For this review, take the finished solid that the model builds, in its own axes (mm). Round coordinates to 2 decimals unless told otherwise and drop trailing zeros. Write each loop counter-clockwise with the first axis right and the second up, starting at its lowest first coordinate (ties: lowest second). Pieces come first, ordered by that corner, then holes. Notation, with made-up numbers: (5, 15.25) - (60, 15.25) arc R27 ccw to (60, 41.25) - close; hole circle Ø3 at (63, -26.5). An arc over 180 degrees is marked (long way). One line per item, written item: value. Start each with the question number.
Q1. Clearance check with flat-ended pins moving along their axes: pin 1 Ø1.5 at (y, z) = (28, 1.5) entering from -X; pin 2 Ø1.5 at (y, z) = (-18, 1) entering from +X; pin 3 Ø0.9 at (y, z) = (79.5, 1.5) entering from -X; pin 4 Ø12 at (x, y) = (-57.5, 5.5) entering from -Z. State where each tip first meets the part, or that it passes through.
Q2. Add section A-A on x = -21. Write out the cut boundary in (y, z).
Q3. For probe 1 along Y at (x, z) = (-22, 0.65); probe 2 along X at (y, z) = (36, 0.7); probe 3 along Y at (x, z) = (23.5, 2.3), list the stretches that pass through material, from the lowest coordinate up.
Q4. Add section C-C on z = 2.15. Give the number of separate pieces and of enclosed holes in the cut face, and give its area (3 significant figures).
Q5. Add section B-B on y = 31.5. Write out the cut boundary in (x, z).
```python
from build123d import *

# Parameters (mm, degrees)
ESQUISSE1_R        = 2.428661445
ESQUISSE1_R_2      = 2.544536974
ESQUISSE1_R_3      = 2.470557968
BOSS_EXTRU_1_DEPTH = 3


with BuildPart() as part:
    # Esquisse1 → Boss.-Extru.1 (new body)
    with BuildSketch(Plane.XY):
        Polygon((-10.741833575, 80.200130208), (19.258166425, 80.200130208), (19.258166425, 77.200130208), (26.258166425, 77.200130208), (26.258166425, 70.200130208), (29.258166425, 70.200130208), (29.258166425, 40.200130208), (26.258166425, 40.200130208), (26.258166425, 20.200130208), (29.258166425, 20.200130208), (29.258166425, -9.799869792), (26.258166425, -9.799869792), (26.258166425, -16.799869792), (19.258166425, -16.799869792), (19.258166425, -19.799869792), (-10.741833575, -19.799869792), (-10.741833575, -16.799869792), (-30.741833575, -16.799869792), (-30.741833575, -19.799869792), (-60.741833575, -19.799869792), (-60.741833575, -16.799869792), (-67.741833575, -16.799869792), (-67.741833575, -9.799869792), (-70.741833575, -9.799869792), (-70.741833575, 20.200130208), (-67.741833575, 20.200130208), (-67.741833575, 40.200130208), (-70.741833575, 40.200130208), (-70.741833575, 70.200130208), (-67.741833575, 70.200130208), (-67.741833575, 77.200130208), (-60.741833575, 77.200130208), (-60.741833575, 80.200130208), (-30.741833575, 80.200130208), (-30.741833575, 77.200130208), (-10.741833575, 77.200130208), align=None)
        with Locations((-20.741833575, 65.411454145)):
            Circle(ESQUISSE1_R, mode=Mode.SUBTRACT)
        with Locations((-20.741833575, 55.962168499)):
            Circle(ESQUISSE1_R_2, mode=Mode.SUBTRACT)
        with Locations((-10.741833575, 55.962168499)):
            Circle(ESQUISSE1_R_3, mode=Mode.SUBTRACT)
    extrude(amount=BOSS_EXTRU_1_DEPTH)


solid = part.part
```
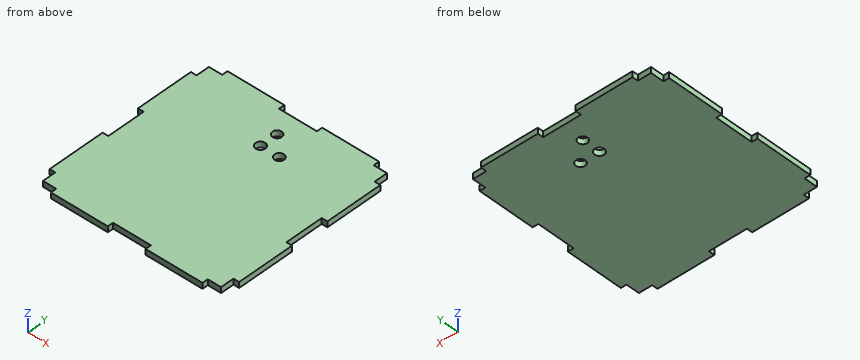
Result set:
1. pin 1: stops at x = -67.74
1. pin 2: stops at x = 19.26
1. pin 3: stops at x = -60.74
1. pin 4: stops at z = 0
2. outline: (-16.8, 0) - (53.43, 0) - (53.43, 3) - (-16.8, 3) - close; (58.49, 0) - (63, 0) - (63, 3) - (58.49, 3) - close; (67.83, 0) - (77.2, 0) - (77.2, 3) - (67.83, 3) - close
3. probe 1: y = -16.8 to 53.75, 58.17 to 63.33, 67.49 to 77.2
3. probe 2: x = -67.74 to 26.26
3. probe 3: y = -16.8 to 77.2
4. separate pieces: 1
4. enclosed holes: 3
4. area: 9,500 mm^2
5. outline: (-67.74, 0) - (26.26, 0) - (26.26, 3) - (-67.74, 3) - close
